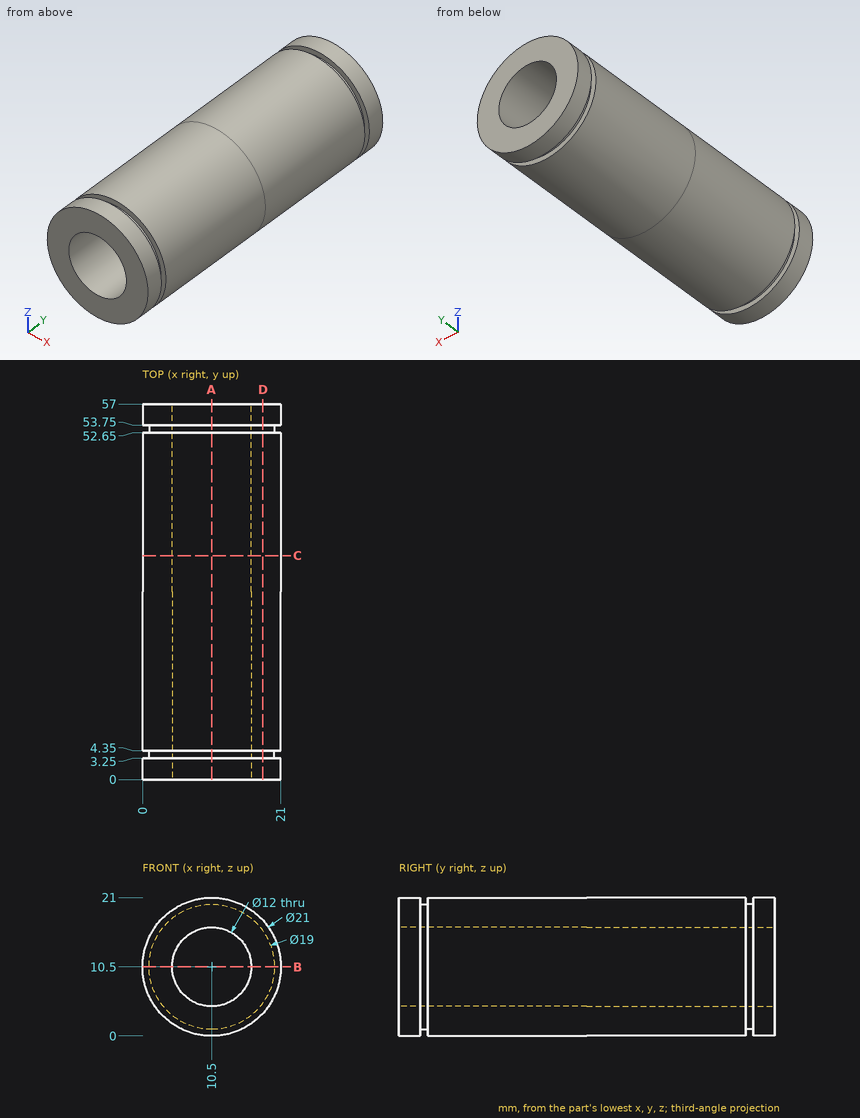
Source: three-view drawing plus pictorial views. Frame: mm from the lowest corner of the part. Round coordinates to 2 decimals unless told otherwise and drop trailing zeros. Write each loop counter-clockwise with the first axis right and the second up, starting at its lowest first coordinate (ties: lowest second). Pieces come first, ordered by that corner, then holes. Notation, with made-up numbers: M 29,-16.75 L 41,-16.75 A11 ccw 41,-8.75 Z; hole C 49.25,29 d8. An arc over 180 degrees is marked long. Write item = value, one per line.
Item 1: Material intervals for line 1 along X through (y, z) = (16.75, 10.5); line 2 along Z through (x, y) = (14, 14); line 3 along X through (y, z) = (38, 9.25), sorted ascending. Write a range as [from, to].
Findings:
line_1 = [0, 4.5], [16.5, 21]
line_2 = [0.6, 5.63], [15.37, 20.4]
line_3 = [0.07, 4.63], [16.37, 20.93]
Item 2: Section query B-B on z = 10.5. Return loops of the section in (x, y).
Findings:
outline = M 0,0 L 4.5,0 L 4.5,57 L 0,57 L 0,53.75 L 1,53.75 L 1,52.65 L 0,52.65 L 0,4.35 L 1,4.35 L 1,3.25 L 0,3.25 Z; M 16.5,0 L 21,0 L 21,3.25 L 20,3.25 L 20,4.35 L 21,4.35 L 21,52.65 L 20,52.65 L 20,53.75 L 21,53.75 L 21,57 L 16.5,57 Z
Item 3: Pin query (flat end, axial travel): P1, Ø3, axis at x = 6.5, y = 18.5, coming from the -Z side; P2, Ø8, axis at y = 19, z = 13.5, coming from the -X side; P3, Ø1, axis at x = 9.5, y = 21.5, coming from the -Z side; P4, Ø10, axis at y = 50.5, z = 18.5, coming from the +X side. Return the tip coordinate at first contact, or that it passes through.
Findings:
P1 = 0.3
P2 = 0
P3 = 0.01
P4 = 20.56
Item 4: Section query D-D on x = 18.25. Return loops of the section in (y, z), then the cut area to 3 significant figures.
Findings:
outline = M 0,3.42 L 3.25,3.42 L 3.25,5.01 L 4.35,5.01 L 4.35,3.42 L 52.65,3.42 L 52.65,5.01 L 53.75,5.01 L 53.75,3.42 L 57,3.42 L 57,17.58 L 53.75,17.58 L 53.75,15.99 L 52.65,15.99 L 52.65,17.58 L 4.35,17.58 L 4.35,15.99 L 3.25,15.99 L 3.25,17.58 L 0,17.58 Z
area = 801 mm^2
Item 5: Section query A-A on x = 10.5. Return loops of the section in (y, z).
Findings:
outline = M 0,0 L 3.25,0 L 3.25,1 L 4.35,1 L 4.35,0 L 52.65,0 L 52.65,1 L 53.75,1 L 53.75,0 L 57,0 L 57,4.5 L 0,4.5 Z; M 0,16.5 L 57,16.5 L 57,21 L 53.75,21 L 53.75,20 L 52.65,20 L 52.65,21 L 4.35,21 L 4.35,20 L 3.25,20 L 3.25,21 L 0,21 Z
Item 6: Section query C-C on y = 34. Return loops of the section in (x, z), then the cut area to 3 significant figures.
Findings:
outline = C 10.5,10.5 d21; hole C 10.5,10.5 d12
area = 233 mm^2
